Part print with two shaded views. Sizes in mm from the minimum x, y, z corner. Give positions to 0.01 mm unless a question says otherwise; leave off trailing zeros. Order: outer loops, then holes, each group sorted by start corner. A loop starts at its lowest first (then second) coordinate and runs counter-clockwise, first axis right, second up. Notation, with made-up numbers: M -22.5,82.25 L -1.5,82.25 A32 cw -1.5,112.25 Z; hole C 67.5,7.5 d4. An arc over 180 degrees is marked long. Return JSON: item names as keys, results as strings. Group by question number.
1. Pin check, flat tips, straight feed: pin 1 (3 mm diameter, centred on x = 13.62, y = 30.5, fed in from +Z); pin 2 (5 mm diameter, centred on x = 13, y = 16.5, fed in from -Z). Stop position of each tip, or through.
2. Wall check: probe 1 along X at (y, z) = (30.5, 2.3); probe 2 along Y at (x, z) = (62.62, 3); probe 3 along Y at (x, z) = (36.5, 4.1) (1 decimal). Give the ranges that are in metal, low to high. Write a range as [from, to].
3. Slice it at A-A on x = 13.62. List the corners of the cut face in (y, z), then the cut area to 3 significant figures.
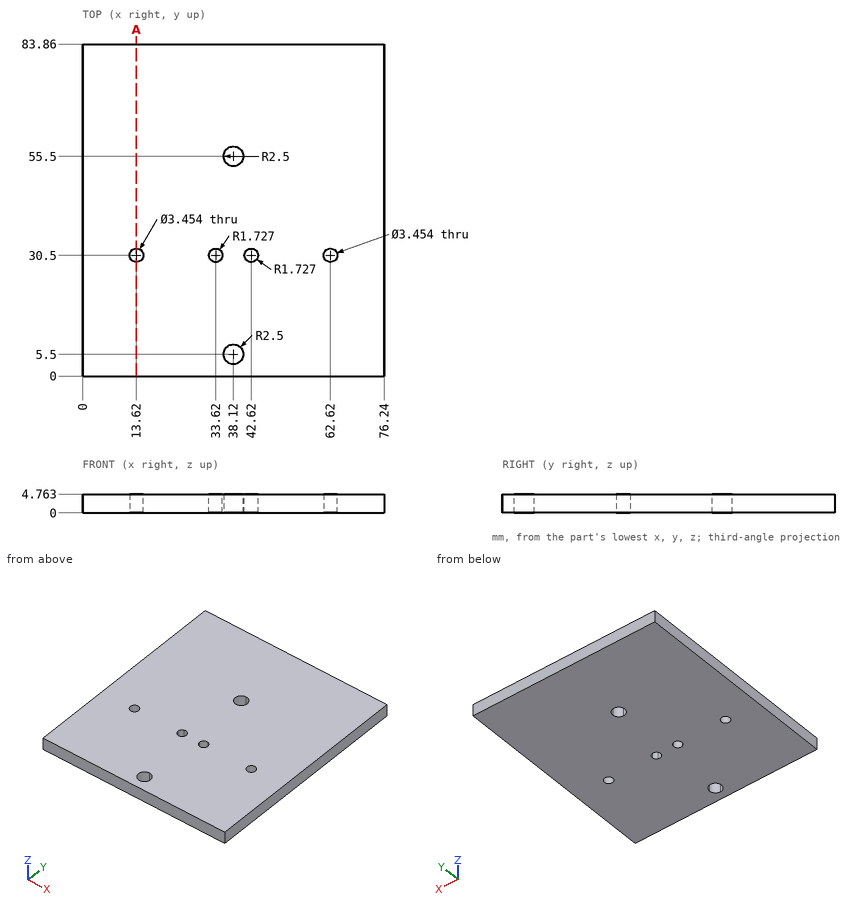
Result:
{
 "1": {"pin 1": "passes through", "pin 2": "stops at z = 0"},
 "2": {"probe 1": "x = [0, 11.89], [15.35, 31.89], [35.35, 40.89], [44.35, 60.89], [64.35, 76.24]", "probe 2": "y = [0, 28.77], [32.23, 83.86]", "probe 3": "y = [0, 3.6], [7.4, 53.6], [57.4, 83.9]"},
 "3": {"outline": "M 0,0 L 28.77,0 L 28.77,4.76 L 0,4.76 Z; M 32.23,0 L 83.86,0 L 83.86,4.76 L 32.23,4.76 Z", "area": "383 mm2"}
}
